The model under review builds one solid part; all positions refer to its coordinate system, in mm. A direction names the side the tool comes from. Give positions to 0.01 mm unless a question says otherwise; leave off trailing zeros. Order: outer loops, then holes, each group sorted by start corner. A loop starts at its lowest first (then second) coordinate and runs counter-clockwise, first axis right, second up. Notation, with made-up numbers: (-35, 70.25) - (-9, 70.25) arc R13 ccw to (-9, 85.25) - close; hole circle Ø8 at (-16.75, 87). An arc over 180 degrees is marked (long way). Put each result on its own line as item: value.
```python
from build123d import *

# Parameters (mm, degrees)
BOSS_EXTRUDE1_DEPTH = 1.5
CHAMFER1_SIZE       = 1
CHAMFER1_SIZE2      = 3.732050808
CHAMFER2_SIZE       = 1
CHAMFER2_SIZE2      = 2.144506921


with BuildPart() as part:
    # Sketch1 → Boss-Extrude1 (new body, symmetric)
    with BuildSketch(Plane(origin=(0, 0, 0), x_dir=(0, 0, -1), z_dir=(1, 0, 0))):
        Polygon((45, 0), (0, 0), (0, 4), (-19, 4), (41, 31), (61, 31), (56, 4), (45, 4), align=None)
    extrude(amount=BOSS_EXTRUDE1_DEPTH, both=True)

    # Chamfer1
    chamfer1_edges = [part.edges().sort_by_distance(p)[0] for p in [
        (-1.5, 17.5, -58.5),
        (1.5, 17.5, -58.5),
    ]]
    chamfer1_side = [part.faces().sort_by_distance(p)[0] for p in [
        (0, 17.5, -58.5),
    ]]
    chamfer(chamfer1_edges, length=CHAMFER1_SIZE, length2=CHAMFER1_SIZE2, reference=chamfer1_side[0])

    # Chamfer2
    chamfer2_edges = [part.edges().sort_by_distance(p)[0] for p in [
        (-1.5, 17.5, -11),
        (1.5, 17.5, -11),
    ]]
    chamfer2_side = [part.faces().sort_by_distance(p)[0] for p in [
        (0, 17.5, -11),
    ]]
    chamfer(chamfer2_edges, length=CHAMFER2_SIZE, length2=CHAMFER2_SIZE2, reference=chamfer2_side[0])


solid = part.part
```
(1) Take a section at D-D, the plane z = 11. Write out the cut boundary in (x, y).
The answers:
outline: (-1.5, 4) - (1.5, 4) - (1.5, 5.25) - (0.5, 7.6) - (-0.5, 7.6) - (-1.5, 5.25) - close
(2) Take a section at C-C, the plane y = 8. Write out the cut boundary in (x, z).
The answers:
outline: (-1.5, -52.95) - (-0.5, -56.74) - (0.5, -56.74) - (1.5, -52.95) - (1.5, 4.89) - (0.5, 10.11) - (-0.5, 10.11) - (-1.5, 4.89) - close
(3) Clearance check with flat-ended pins moving along their axes: pin 1 Ø1.5 at (x, z) = (0.5, -33) entering from +Y; pin 2 Ø1 at (x, z) = (-0.5, 11) entering from +Y (3 decimals); pin 3 Ø0.9 at (x, z) = (0, -52) entering from -Y. State where each tip first meets the part, or that it passes through.
The answers:
pin 1: y = 27.74
pin 2: y = 7.825
pin 3: y = 4
(4) Take a section at B-B, the plane z = -24. Write out the cut boundary in (x, y).
The answers:
outline: (-1.5, 0) - (1.5, 0) - (1.5, 21) - (0.5, 23.35) - (-0.5, 23.35) - (-1.5, 21) - close
(5) Take a section at A-A, the plane y = 24.5. Write out the cut boundary in (x, z), then the cut area to 3 significant figures.
The answers:
outline: (-1.5, -56) - (-0.5, -59.8) - (0.5, -59.8) - (1.5, -56) - (1.5, -31.78) - (0.5, -26.56) - (-0.5, -26.56) - (-1.5, -31.78) - close
area: 90.7 mm^2
(6) For faces 1 (the flat face through (0.01, 17.31, -10.58)), 2 (the flat face through (0, 4, 9)), 3 (the flat face through (0, 2, -45)), list the 3-axis set-ups (+Z, -Z, +X, -X, +Y, -Y) from which the entire face can be reached by the end or side of a thin tool; tool diameter is ignored.
The answers:
face 1: +Z, +X, -X, +Y
face 2: +Z, +X, -X, -Y
face 3: -Z, +X, -X, -Y
(7) Wall thickness on L1, parallel to Y at x = 0, z = -46.5; L2, parallel to Y at x = 0.9, z = -18.5; L3, parallel to Z at x = 0.45, y = 19: over which ranges is each line inside the solid? List them lowest first.
The answers:
L1: 4 to 31
L2: 0 to 19.93
L3: -58.78 to -14.33
